from build123d import *

# Parameters (mm, degrees)
SKETCH1_R           = 5
BOSS_EXTRUDE1_DEPTH = 7.5
SKETCH2_R           = 6.35
CUT_EXTRUDE1_DEPTH  = 20


with BuildPart() as part:
    # Sketch1 → Boss-Extrude1 (new body, symmetric)
    with BuildSketch(Plane.XY):
        with BuildLine():
            Line((0, 15), (30, 15))
            Line((30, 15), (30, -15))
            Line((30, -15), (0, -15))
            ThreePointArc((0, -15), (-15, 0), (0, 15))
        make_face()
        Circle(SKETCH1_R, mode=Mode.SUBTRACT)
    extrude(amount=BOSS_EXTRUDE1_DEPTH, both=True)

    # Sketch2 → Cut-Extrude1 (cut)
    with BuildSketch(Plane(origin=(30, 0, 0), x_dir=(0, 0, -1), z_dir=(1, 0, 0))):
        Circle(SKETCH2_R)
    extrude(amount=-CUT_EXTRUDE1_DEPTH, mode=Mode.SUBTRACT)


solid = part.part
Geometry check sheet. Reference: the model listing, model coordinates, mm. A direction names the side the tool comes from. Give positions to 0.01 mm unless a question says otherwise; leave off trailing zeros. Loops run counter-clockwise (first coordinate to the right, second up) from the corner with the lowest first, then second, coordinate; pieces in that order, holes last. Notation, with made-up numbers: M 68.25,58 L 104.25,58 A7 ccw 104.25,71 Z; hole C 7.25,-7 d6. An arc over 180 degrees is marked long. Answer as a JSON object with one key per item and string values. Group by question number.
Item 1: Gauge pin test, flat ends, axial feed: pin 1 (3 mm diameter, centred on x = -10.5, z = 4, fed in from -Y); pin 2 (2 mm diameter, centred on y = -9, z = -2, fed in from -X); pin 3 (1 mm diameter, centred on y = 5.5, z = 0.5, fed in from -X). Record the tip position at first contact, or that the pin passes through.
Item 2: Sectioned sample at B-B on x = 3. Record the boundary of the cut face in (y, z).
Item 3: Material ranges on L1, parallel to Y at x = 0, z = 2.25; L2, parallel to Y at x = 20.25, z = 0; L3, parallel to X at y = 1.5, z = 4.25, recorded low to high.
Item 4: Sectioned sample at C-C on z = 0. Record the boundary of the cut face in (x, y).
Item 5: Mould release check, pull along Z, two halves, no side actions. Record for faces 3 (the cylindrical face through (20.14, -6.2, 1.38)), 4 (the flat face through (8, 0, -7.5)), 5 (the flat face through (15, 15, 0)): pulls with the +Z half, pulls with the -Z half, needs draft (parallel to the pull), parting line crosses it, or undercut.
Item 6: Sectioned sample at D-D on x = 15. Record the boundary of the cut face in (y, z).
Item 7: Sectioned sample at A-A on y = 0. Record the boundary of the cut face in (x, z).
Item 8: Access from +Z, -Z, +X, -X, +Y, -Y to the whole of each face (thin tool, end or side, straight path). Record for faces 1 (the flat face through (10, 0, 0)), 2 (the cylindrical face through (-15, 0, 0)).
Findings below:
{
 "1": {"pin 1": "y = -12", "pin 2": "x = -12.69", "pin 3": "x = -14.14"},
 "2": {"outline": "M -15,-7.5 L -4,-7.5 L -4,7.5 L -15,7.5 Z; M 4,-7.5 L 15,-7.5 L 15,7.5 L 4,7.5 Z"},
 "3": {"L1": "-15 to -5, 5 to 15", "L2": "-15 to -6.35, 6.35 to 15", "L3": "-14.92 to -4.77, 4.77 to 10"},
 "4": {"outline": "M 0,-15 L 30,-15 L 30,-6.35 L 10,-6.35 L 10,6.35 L 30,6.35 L 30,15 L 0,15 A15 ccw Z; hole C 0,0 d10"},
 "5": {"face 3": "undercut", "face 4": "pulls with the -Z half", "face 5": "needs draft"},
 "6": {"outline": "M -15,-7.5 L 15,-7.5 L 15,7.5 L -15,7.5 Z; hole C 0,0 d12.7"},
 "7": {"outline": "M -15,-7.5 L -5,-7.5 L -5,7.5 L -15,7.5 Z; M 5,-7.5 L 30,-7.5 L 30,-6.35 L 10,-6.35 L 10,6.35 L 30,6.35 L 30,7.5 L 5,7.5 Z"},
 "8": {"face 1": "+X", "face 2": "+Z, -Z, -X"}
}
